Check sheet for the drawn part. Datum: minimum x, y, z corner. Units: mm. Round coordinates to 2 decimals unless told otherwise and drop trailing zeros. Order: outer loops, then holes, each group sorted by start corner. A loop starts at its lowest first (then second) coordinate and runs counter-clockwise, first axis right, second up. Notation, with made-up numbers: (83.25, -37.5) -> (126.25, -37.5) arc R26 cw to (126.25, -4.5) -> close; hole circle Ø1 at (-35, 58.25). An arc over 180 degrees is marked (long way). Answer in a Markdown table with one row per item.
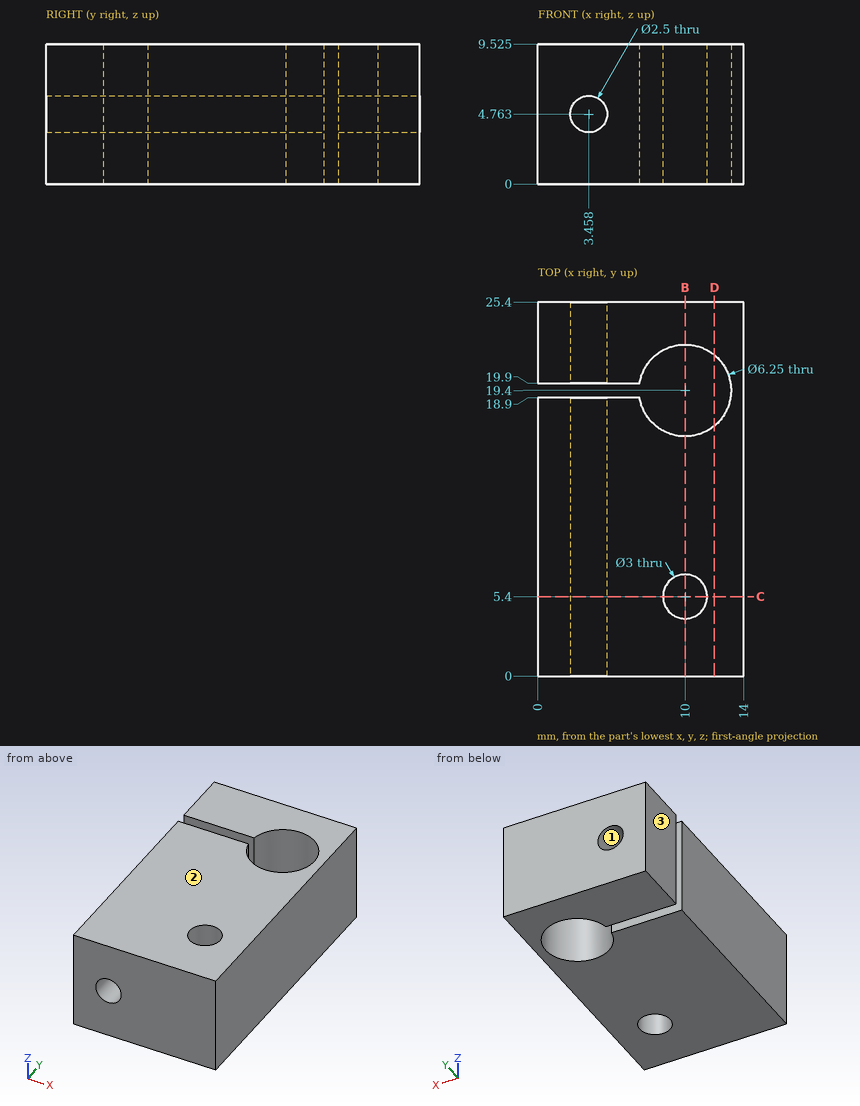
(1) Section check C-C on y = 5.4. Give the number of separate pieces and of enclosed holes in the cut face.
Solutions:
| item | result |
|---|---|
| separate pieces | 2 |
| enclosed holes | 1 |
(2) Draft check along X on the marked faces 1, 2 and 3. Enter one of: pulls with the +X half, pulls with the -X half, needs draft (parallel to the pull), parting line crosses it, or undercut.
Solutions:
| item | result |
|---|---|
| face 1 | undercut |
| face 2 | needs draft |
| face 3 | pulls with the -X half |
(3) Scan lines: probe 1 along Y at (x, z) = (10, 5) (1 decimal); probe 2 along Y at (x, z) = (1.25, 6.5); probe 3 along Y at (x, z) = (9.5, 8.25) (1 decimal). Record each from-to range of solid material in increasing order. Write a range as from..to.
Solutions:
| item | result |
|---|---|
| probe 1 | 0..3.9, 6.9..16.3, 22.5..25.4 |
| probe 2 | 0..18.9, 19.9..25.4 |
| probe 3 | 0..4, 6.8..16.3, 22.5..25.4 |
(4) Section check D-D on x = 12. Record the boundary of the cut face in (y, z) (1 decimal).
Solutions:
| item | result |
|---|---|
| outline | (0, 0) -> (17, 0) -> (17, 9.5) -> (0, 9.5) -> close; (21.8, 0) -> (25.4, 0) -> (25.4, 9.5) -> (21.8, 9.5) -> close |
(5) Section check B-B on x = 10. Record the boundary of the cut face in (y, z) (1 decimal), plus the area to 3 significant figures.
Solutions:
| item | result |
|---|---|
| outline | (0, 0) -> (3.9, 0) -> (3.9, 9.5) -> (0, 9.5) -> close; (6.9, 0) -> (16.3, 0) -> (16.3, 9.5) -> (6.9, 9.5) -> close; (22.5, 0) -> (25.4, 0) -> (25.4, 9.5) -> (22.5, 9.5) -> close |
| area | 154 mm^2 |
